Part print with two shaded views. Sizes in mm from the minimum x, y, z corner. A direction names the side the tool comes from. Round coordinates to 2 decimals unless told otherwise and drop trailing zeros. Loops run counter-clockwise (first coordinate to the right, second up) from the corner with the lowest first, then second, coordinate; pieces in that order, holes last. Notation, with made-up numbers: (14.25, 35) -> (70.25, 35) arc R31 cw to (70.25, 60) -> close; hole circle Ø8 at (47, -13). An arc over 180 degrees is marked (long way). Put each result on its own line as item: value. Start each with the question number.
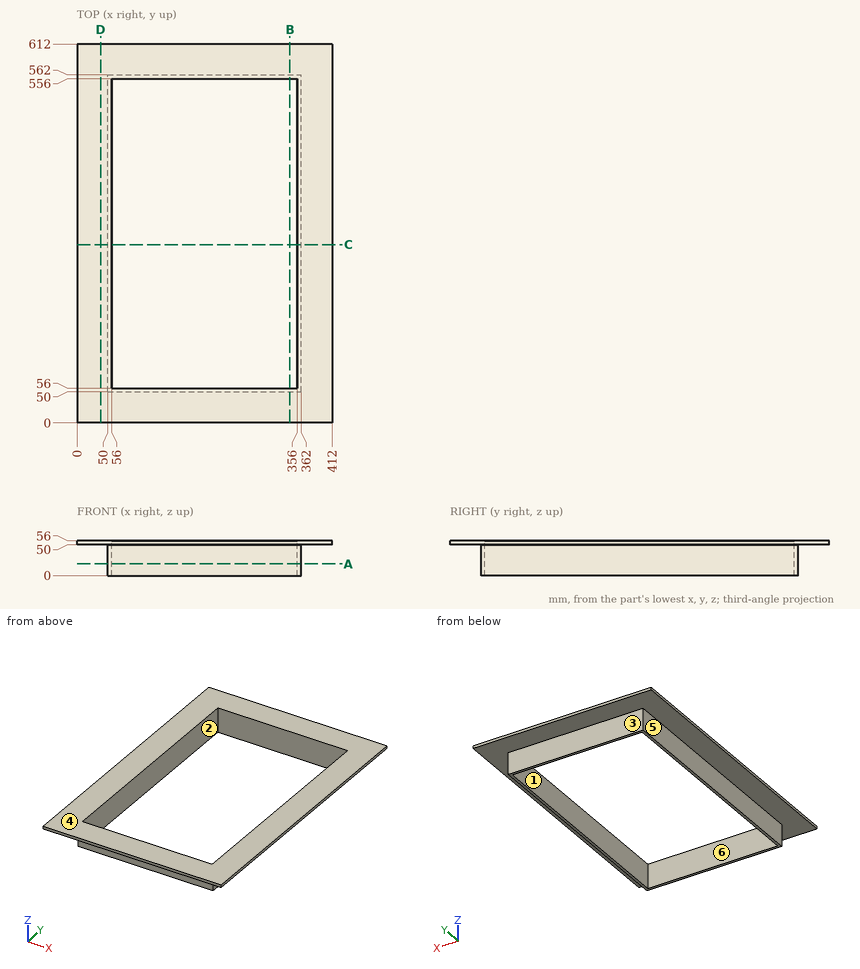
Item 1: Wall check: line 1 (Y direction, x = 173, z = 18.5); line 2 (X direction, y = 525.5, z = 16.5); line 3 (Z direction, x = 49, y = 73). Give the ranges that are in metal, low to high. Write a range as from..to.
Item 2: Pull direction Y, two halves, no side cores. Call the marked faces 1, 2, 3 and 4: +Y half, -Y half, draft (parallel to the pull), parting line (faces both ways), or undercut.
Item 3: Cut at A-A on z = 19. Write the cut outline in (x, y), then the cut area to 3 significant figures.
Item 4: 3-axis set-ups, long thin cutter, end or side, ignore diameter. For the marked faces 5 and 6: which of +Z, -Z, +X, -X, +Y, -Y reach the whole face in a straight line?
Item 5: Drop flat-ended pins along their axis: pin 1 (1.5 mm diameter, centred on x = 101.5, z = 22.5, fed in from -Y); pin 2 (3 mm diameter, centred on y = 342.5, z = 20.5, fed in from -X); pin 3 (1.5 mm diameter, centred on x = 343, z = 15.5, fed in from +Y). Give the stop position or say it passes through.
Item 6: Cut at D-D on x = 38. Write the cut outline in (y, z).
Item 7: Cut at C-C on y = 288. Write the cut outline in (x, z), then the cut area to 3 significant figures.
Item 8: Cut at B-B on x = 344. Write the cut outline in (y, z), then the cut area to 3 significant figures.
Ans:
1. line 1: y = 50..56, 556..562
1. line 2: x = 50..56, 356..362
1. line 3: z = 50..56
2. face 1: undercut
2. face 2: undercut
2. face 3: +Y half
2. face 4: draft
3. outline: (50, 50) -> (362, 50) -> (362, 562) -> (50, 562) -> close; hole (56, 56) -> (356, 56) -> (356, 556) -> (56, 556) -> close
3. area: 9,740 mm2
4. face 5: -Z, -X, +Y, -Y
4. face 6: +Z, -Z
5. pin 1: stops at y = 50
5. pin 2: stops at x = 50
5. pin 3: stops at y = 562
6. outline: (0, 50) -> (612, 50) -> (612, 56) -> (0, 56) -> close
7. outline: (0, 50) -> (50, 50) -> (50, 0) -> (56, 0) -> (56, 56) -> (0, 56) -> close; (356, 0) -> (362, 0) -> (362, 50) -> (412, 50) -> (412, 56) -> (356, 56) -> close
7. area: 1,270 mm2
8. outline: (0, 50) -> (50, 50) -> (50, 0) -> (56, 0) -> (56, 56) -> (0, 56) -> close; (556, 0) -> (562, 0) -> (562, 50) -> (612, 50) -> (612, 56) -> (556, 56) -> close
8. area: 1,270 mm2
